Part model, mm, in its own coordinate system. A direction names the side the tool comes from. Give positions to 0.01 mm unless a question says otherwise; leave off trailing zeros. Write each loop counter-clockwise with the first axis right and the second up, starting at its lowest first coordinate (ties: lowest second). Pieces come first, ordered by that corner, then holes. Notation, with made-up numbers: (-25.75, 44.25) - (30.25, 44.25) arc R21 ccw to (30.25, 57.25) - close; hole circle Ø4 at (-39, 67). An arc over 180 degrees is marked (long way). Answer in a Markdown table with one row per item. Add a question column.
1. Band-saw the part on B-B on z = 27.5. Write the cut outline in (x, y), plus the area to 3 significant figures.
2. Band-saw the part on A-A on y = -14.5. Write the cut outline in (x, z).
3. Which spindle directions (+Z, -Z, +X, -X, +Y, -Y) get a long thin tool onto all of the face, cutting with end or side? Do faces 1 (the flat face through (-4, -17, 12.7)), 2 (the flat face through (19, 1.846, 12)), 3 (the flat face through (38.8, -13.9, 12.7)). Say none if no direction does.
4. Probe line 1 along Z through (x, y) = (8.5, -10.5); line 2 along X through (y, z) = (-17.25, 29.5); line 3 along Y through (x, z) = (24, 34). List the from-to ranges inside material, lowest first.
5. Band-saw the part on C-C on x = -10. Write the cut outline in (y, z).
6. Pull direction Y, two halves, no side cores. Call faces 4 (the cylindrical face through (38.263, -10.575, 6.439)), 5 (the flat face through (19, -23.554, 12)), 6 (the flat face through (6.507, -11, 25)): released by +Y, released by -Y, zero draft, split by the parting line, or undercut.
7. Drop flat-ended pins along their axis: pin 1 Ø2 at (x, z) = (22, 38.5) entering from +Y; pin 2 Ø6 at (x, y) = (22.5, -5.5) entering from +Z; pin 3 Ø5 at (x, y) = (-1.5, -3) entering from +Z; pin 4 Ø12 at (x, y) = (-9.5, -1.5) entering from -Z. Give the stop position or say it passes through.
8. Band-saw the part on D-D on x = 31. Write the cut outline in (y, z), plus the area to 3 significant figures.
```python
from build123d import *

# Parameters (mm, degrees)
F0_W      = 76.2
F0_H      = 25.4
F1_DEPTH  = 44.45
F2_W      = 25.4
F2_H      = 31.75
F3_DEPTH  = 25.4
F4_R      = 6.35
F5_DEPTH  = 25.4
F7_DEPTH  = 25.4
F9_DEPTH  = 25.4
F11_DEPTH = 25.4
F13_DEPTH = 25.4
F15_DEPTH = 25.4


with BuildPart() as f1:
    # F0 (on Top) → F1 (new body)
    with BuildSketch(Plane.XY):
        with Locations((19.2070399102, -10.8540700749)):
            Rectangle(F0_W, F0_H)
    extrude(amount=F1_DEPTH)

    # F2 (on face) → F3 (cut)
    with BuildSketch(Plane.XZ.offset(23.5540700749)):
        with Locations((-6.1929600898, 28.575)):
            Rectangle(F2_W, F2_H)
        with Locations((44.6070399102, 28.575)):
            Rectangle(F2_W, F2_H)
    extrude(amount=-F3_DEPTH, mode=Mode.SUBTRACT)

    # F4 (on face) → F5 (cut)
    with BuildSketch(Plane.XY.offset(12.7)):
        with Locations((44.6070399102, -10.8540700749)):
            Circle(F4_R)
    extrude(amount=-F5_DEPTH, mode=Mode.SUBTRACT)

    # F6 (on face) → F7 (cut)
    with BuildSketch(Plane.XY.offset(12.7)):
        with BuildLine():
            ThreePointArc((-6.1929600898, -4.5040700749), (-10.6830881503, -15.3441981354), (0.1570399102, -10.8540700749))
            ThreePointArc((0.1570399102, -10.8540700749), (-1.7028320292, -6.3639420143), (-6.1929600898, -4.5040700749))
        make_face()
    extrude(amount=-F7_DEPTH, mode=Mode.SUBTRACT)

    # F8 (on face) → F9 (cut)
    with BuildSketch(Plane.XY.offset(12.7)):
        with BuildLine():
            ThreePointArc((44.6070399102, 1.8459299251), (53.5872960313, -1.8738139538), (57.3070399102, -10.8540700749))
            Line((57.3070399102, -10.8540700749), (57.3070399102, 1.8459299251))
            Line((57.3070399102, 1.8459299251), (44.6070399102, 1.8459299251))
        make_face()
        with BuildLine():
            ThreePointArc((57.3070399102, -10.8540700749), (53.5872960313, -19.8343261959), (44.6070399102, -23.5540700749))
            Line((44.6070399102, -23.5540700749), (57.3070399102, -23.5540700749))
            Line((57.3070399102, -23.5540700749), (57.3070399102, -10.8540700749))
        make_face()
    extrude(amount=-F9_DEPTH, mode=Mode.SUBTRACT)

    # F10 (on face) → F11 (cut)
    with BuildSketch(Plane.XY.offset(12.7)):
        with BuildLine():
            ThreePointArc((-6.1929600898, -23.5540700749), (-15.173216183, -19.8343262238), (-18.8929600898, -10.8540701536))
            Line((-18.8929600898, -10.8540701536), (-18.8929600898, -23.5540700749))
            Line((-18.8929600898, -23.5540700749), (-6.1929600898, -23.5540700749))
        make_face()
        with BuildLine():
            ThreePointArc((-18.8929600898, -10.8540701536), (-15.1732162387, -1.8738139816), (-6.1929600898, 1.8459299251))
            Line((-6.1929600898, 1.8459299251), (-18.8929600898, 1.8459299251))
            Line((-18.8929600898, 1.8459299251), (-18.8929600898, -10.8540701536))
        make_face()
    extrude(amount=-F11_DEPTH, mode=Mode.SUBTRACT)

    # F12 (on face) → F13 (cut)
    with BuildSketch(Plane.YZ.offset(31.9070399102)):
        with BuildLine():
            Line((-4.5040700749, 31.75), (-17.2040700749, 31.75))
            ThreePointArc((-17.2040700749, 31.75), (-10.8540700749, 25.4), (-4.5040700749, 31.75))
        make_face()
        with BuildLine():
            ThreePointArc((-4.5040700749, 31.75), (-10.8540700749, 38.1), (-17.2040700749, 31.75))
            Line((-17.2040700749, 31.75), (-4.5040700749, 31.75))
        make_face()
    extrude(amount=-F13_DEPTH, mode=Mode.SUBTRACT)

    # F14 (on face) → F15 (cut)
    with BuildSketch(Plane.YZ.offset(31.9070399102)):
        with BuildLine():
            ThreePointArc((-23.5540700749, 31.75), (-19.8343261959, 40.7302561211), (-10.8540700749, 44.45))
            Line((-10.8540700749, 44.45), (-23.5540700749, 44.45))
            Line((-23.5540700749, 44.45), (-23.5540700749, 31.75))
        make_face()
        with BuildLine():
            ThreePointArc((-10.8540700749, 44.45), (-1.8738139538, 40.7302561211), (1.8459299251, 31.75))
            Line((1.8459299251, 31.75), (1.8459299251, 44.45))
            Line((1.8459299251, 44.45), (-10.8540700749, 44.45))
        make_face()
    extrude(amount=-F15_DEPTH, mode=Mode.SUBTRACT)


solid = f1.part
```
Values:
| question | item | result |
|---|---|---|
| 1 | outline | (6.51, -23.55) - (31.91, -23.55) - (31.91, -15.57) - (6.51, -15.57) - close; (6.51, -6.14) - (31.91, -6.14) - (31.91, 1.85) - (6.51, 1.85) - close |
| 1 | area | 405 mm² |
| 2 | outline | (-18.36, 0) - (-11.39, 0) - (-11.39, 12.7) - (-18.36, 12.7) - close; (-0.99, 0) - (39.41, 0) - (39.41, 12.7) - (31.91, 12.7) - (31.91, 26.55) - (6.51, 26.55) - (6.51, 12.7) - (-0.99, 12.7) - close; (6.51, 36.95) - (31.91, 36.95) - (31.91, 43.92) - (6.51, 43.92) - close; (49.81, 0) - (56.77, 0) - (56.77, 12.7) - (49.81, 12.7) - close |
| 3 | face 1 | +Z, -X, +Y, -Y |
| 3 | face 2 | +Z, -Z, +X, -X, +Y |
| 3 | face 3 | +Z, +X, +Y, -Y |
| 4 | line 1 | z = 0 to 25.41, 38.09 to 44.45 |
| 4 | line 2 | x = 6.51 to 31.91 |
| 4 | line 3 | y = -23.35 to -16.79, -4.92 to 1.65 |
| 5 | outline | (-22.97, 0) - (-15.94, 0) - (-15.94, 12.7) - (-22.97, 12.7) - close; (-5.77, 0) - (1.26, 0) - (1.26, 12.7) - (-5.77, 12.7) - close |
| 6 | face 4 | undercut |
| 6 | face 5 | released by -Y |
| 6 | face 6 | zero draft |
| 7 | pin 1 | stops at y = 0.47 |
| 7 | pin 2 | stops at z = 44.23 |
| 7 | pin 3 | stops at z = 12.7 |
| 7 | pin 4 | stops at z = 0 |
| 8 | outline | (-23.55, 0) - (1.85, 0) - (1.85, 31.75) arc R12.7 ccw to (-23.55, 31.75) - close; hole circle Ø12.7 at (-10.85, 31.75) |
| 8 | area | 933 mm² |
